```python
from build123d import *

# Parameters (mm, degrees)
SHELL1_T            = -4
FILLET1_R           = 10
BOSS_EXTRUDE4_DEPTH = 200
CUT_EXTRUDE1_DEPTH  = 200
FILLET3_R           = 2


with BuildPart() as part:
    # Sketch3 for Loft1 → Loft1 section 0
    with BuildSketch(Plane(origin=(0, 200, 0), x_dir=(1, 0, 0), z_dir=(0, 1, 0))):
        with BuildLine():
            Line((-91.643479102, 47.875432933), (48.356520898, 47.875432933))
            Line((48.356520898, 47.875432933), (48.356520898, -5.122491685))
            # circular arc as an exact rational Bezier (weights 1, cos(half-angle), 1)
            Bezier((48.356520898, -5.122491685), (48.356520898, -12.124567067), (41.776722331, -14.519417892), weights=[1, 0.819152044, 1])
            Line((41.776722331, -14.519417892), (-20.959438815, -37.353513162))
            Bezier((-20.959438815, -37.353513162), (-21.643479102, -37.602483465), (-22.327519388, -37.353513162), weights=[1, 0.939692621, 1])
            Line((-22.327519388, -37.353513162), (-85.063680535, -14.519417892))
            Bezier((-85.063680535, -14.519417892), (-91.643479102, -12.124567067), (-91.643479102, -5.122491685), weights=[1, 0.819152044, 1])
            Line((-91.643479102, -5.122491685), (-91.643479102, 47.875432933))
        make_face()
    # Sketch2 for Loft1 → Loft1 section 1
    with BuildSketch(Plane(origin=(0, 0, 0), x_dir=(1, 0, 0), z_dir=(0, 1, 0))):
        with BuildLine():
            Line((-91.643479102, 47.875432933), (48.356520898, 47.875432933))
            Line((48.356520898, 47.875432933), (48.356520898, -5.122491685))
            Bezier((48.356520898, -5.122491685), (48.356520898, -12.124567067), (41.776722331, -14.519417892), weights=[1, 0.819152044, 1])
            Line((41.776722331, -14.519417892), (-20.959438815, -37.353513162))
            Bezier((-20.959438815, -37.353513162), (-21.643479102, -37.602483465), (-22.327519388, -37.353513162), weights=[1, 0.939692621, 1])
            Line((-22.327519388, -37.353513162), (-85.063680535, -14.519417892))
            Bezier((-85.063680535, -14.519417892), (-91.643479102, -12.124567067), (-91.643479102, -5.122491685), weights=[1, 0.819152044, 1])
            Line((-91.643479102, -5.122491685), (-91.643479102, 47.875432933))
        make_face()
    loft()

    # Shell1
    shell1_openings = [part.faces().sort_by_distance(p)[0] for p in [
        (-21.643479102, 0, -11.173558068),
        (-21.643479102, 200, -11.173558068),
    ]]
    offset(amount=SHELL1_T, openings=shell1_openings)

    # Fillet1
    fillet1_edges = [part.edges().sort_by_distance(p)[0] for p in [
        (-21.643479102, 100, 33.345772375),
    ]]
    fillet(fillet1_edges, radius=FILLET1_R)

    # Sketch7 → Boss-Extrude4 (add)
    with BuildSketch(Plane(origin=(0, 200, 0), x_dir=(1, 0, 0), z_dir=(0, 1, 0))):
        Polygon((46.356653815, -4.610276577), (46.356653815, -9.110276577), (31.356653815, -14.569830091), (31.356653815, -4.610276577), align=None)
        Polygon((-89.643479632, -4.610276577), (-89.643479632, -9.110276577), (-74.643479632, -14.569830091), (-74.643479632, -4.610276577), align=None)
    extrude(amount=-BOSS_EXTRUDE4_DEPTH)

    # Sketch8 → Cut-Extrude1 (cut)
    with BuildSketch(Plane(origin=(0, 200, 0), x_dir=(1, 0, 0), z_dir=(0, 1, 0))):
        Polygon((-87.643479102, 47.875432933), (-77.643479102, 47.875432933), (34.356520898, 47.875432933), (44.356520898, 47.875432933), (44.356520898, 45.875432933), (34.356520898, 45.875432933), (34.356520898, 43.875432933), (-77.643479102, 43.875432933), (-77.643479102, 45.875432933), (-87.643479102, 45.875432933), align=None)
    extrude(amount=-CUT_EXTRUDE1_DEPTH, mode=Mode.SUBTRACT)

    # Fillet3
    fillet3_edges = [part.edges().sort_by_distance(p)[0] for p in [
        (44.356520898, 100, -43.875432933),
        (-87.643479102, 100, -43.875432933),
    ]]
    fillet(fillet3_edges, radius=FILLET3_R)


solid = part.part
```
For this review, take the finished solid that the model builds, in its own axes (mm). A direction names the side the tool comes from. Coordinates: 2 decimals unless noted, no trailing zeros. Order: outer loops, then holes, each group sorted by start corner. A loop starts at its lowest first (then second) coordinate and runs counter-clockwise, first axis right, second up. Notation, with made-up numbers: (-16.75, -35.5) - (3.25, -35.5) arc R7 ccw to (3.25, -22.5) - close; hole circle Ø10 at (29, 16.5). An arc over 180 degrees is marked (long way). Answer as a JSON object with one key per item and string values. Group by question number.
1. For probe 1 along X at (y, z) = (101, -15.5); probe 2 along Z at (x, y) = (-21, 165.5); probe 3 along X at (y, z) = (57.5, 7), list the stretches that pass through material, from the lowest coordinate up.
2. The part is to be moulded in two halves that separate along Z. For faces 4 (the flat face through (46, 99, -47.875)), 5 (the flat face through (44.357, 99, -19)), 6 (the flat face through (-74.643, 101, 9)), say which applies: pulls with the +Z half, pulls with the -Z half, needs draft (parallel to the pull), parting line crosses it, or undercut.
3. Clearance check with flat-ended pins moving along their axes: P1, Ø5, axis at x = -83, y = 106, coming from the -Z side; P2, Ø7.5, axis at y = 110.5, z = 9.5, coming from the +X side; P3, Ø6, axis at x = 4, y = 149, coming from the -Z side. State where each tip first meets the part, or that it passes through.
4. We need section C-C on x = 2. State the section outline as (y, z) points, then the cut area to 3 significant figures.
5. For faces 1 (the flat face through (31.357, 101, 9)), 2 (the flat face through (38, 99, -43.875)), 3 (the flat face through (-12, 200, 31)), list the 3-axis set-ups (+Z, -Z, +X, -X, +Y, -Y) from which the entire face can be reached by the end or side of a thin tool; tool diameter is ignored.
6. We need section B-B on z = 30. State the section outline as (x, y) points, then the cut area to 3 significant figures.
7. We need section A-A on z = -1. State the section outline as (x, y) points, then the cut area to 3 significant figures.
Final values:
{
 "1": {"probe 1": "-91.64 to -87.64, 44.36 to 48.36", "probe 2": "32.68 to 37.37", "probe 3": "-91.47 to -74.64, 31.36 to 48.18"},
 "2": {"face 4": "pulls with the -Z half", "face 5": "undercut", "face 6": "needs draft"},
 "3": {"P1": "z = -45.88", "P2": "x = 48.34", "P3": "z = 22.92"},
 "4": {"outline": "(0, 24.74) - (200, 24.74) - (200, 29) - (0, 29) - close", "area": "851 mm²"},
 "5": {"face 1": "-Z, +Y, -Y", "face 2": "+Y, -Y", "face 3": "+Z, -Z, +X, -X, +Y"},
 "6": {"outline": "(-42.53, 0) - (-30.84, 0) - (-30.84, 200) - (-42.53, 200) - close; (-12.45, 0) - (-0.76, 0) - (-0.76, 200) - (-12.45, 200) - close", "area": "4,680 mm²"},
 "7": {"outline": "(-91.64, 0) - (-87.64, 0) - (-87.64, 200) - (-91.64, 200) - close; (44.36, 0) - (48.36, 0) - (48.36, 200) - (44.36, 200) - close", "area": "1,600 mm²"}
}
